```python
from build123d import *
from build123d.topology import SkipClean

# Parameters (mm, degrees)
SKETCH1_R                    = 4
COUPLER_SECTION_DEPTH        = 12.5
SKETCH3_R                    = 5
BEARING_SECTION_DEPTH        = 12
SKETCH4_R                    = 7
BEARING_STOP_DEPTH           = 3
SKETCH5_R                    = 4
SMALL_SEAL_SECTION_DEPTH     = 12.3
SET_SCREW_FLAT_SECTION_DEPTH = 10.5
SKETCH7_R                    = 4
IMPELLER_SECTION_DEPTH       = 15.35455
SKETCH8_R                    = 1.5
IMPELLER_BOLT_BORE_DEPTH     = 8
DOWEL_PIN_HOLE_DEPTH         = 23
DOWEL_PIN_HOLE_DEPTH_BACK    = 23
SKETCH9_R                    = 1


with BuildPart() as part:
    # Sketch1 → coupler section (new body)
    with BuildSketch(Plane(origin=(0, 0, 0), x_dir=(1, 0, 0), z_dir=(0, 1, 0))):
        with Locations(Location((0, 0, 0), (0, 0, 270))):
            Circle(SKETCH1_R)
    extrude(amount=COUPLER_SECTION_DEPTH)

    # Sketch3 → bearing section (add)
    with BuildSketch(Plane(origin=(0, 12.5, 0), x_dir=(1, 0, 0), z_dir=(0, 1, 0))):
        with Locations(Location((0, 0, 0), (0, 0, 270))):
            Circle(SKETCH3_R)
    extrude(amount=BEARING_SECTION_DEPTH)

    # Sketch4 → bearing stop (add)
    with BuildSketch(Plane(origin=(0, 24.5, 0), x_dir=(1, 0, 0), z_dir=(0, 1, 0))):
        with Locations(Location((0, 0, 0), (0, 0, 270))):
            Circle(SKETCH4_R)
    extrude(amount=BEARING_STOP_DEPTH)

    # Sketch5 → small seal section (add)
    with BuildSketch(Plane(origin=(0, 27.5, 0), x_dir=(1, 0, 0), z_dir=(0, 1, 0))):
        with Locations(Location((0, 0, 0), (0, 0, 270))):
            Circle(SKETCH5_R)
    extrude(amount=SMALL_SEAL_SECTION_DEPTH)

    # Sketch6 → set screw flat section (cut)
    with BuildSketch(Plane.XZ):
        with BuildLine():
            Line((-2.645751311, 3), (2.645751311, 3))
            ThreePointArc((2.645751311, 3), (0, 4), (-2.645751311, 3))
        make_face()
    extrude(amount=-SET_SCREW_FLAT_SECTION_DEPTH, mode=Mode.SUBTRACT)

    # Sketch7 → impeller section (add)
    with BuildSketch(Plane(origin=(0, 39.8, 0), x_dir=(1, 0, 0), z_dir=(0, 1, 0))):
        with Locations(Location((0, 0, 0), (0, 0, 311.409622109))):
            Circle(SKETCH7_R)
    extrude(amount=IMPELLER_SECTION_DEPTH)

    # Sketch8 → impeller bolt bore (cut)
    with BuildSketch(Plane(origin=(0, 55.15455, 0), x_dir=(1, 0, 0), z_dir=(0, 1, 0))):
        with Locations(Location((0, 0, 0), (0, 0, 270))):
            Circle(SKETCH8_R)
    extrude(amount=-IMPELLER_BOLT_BORE_DEPTH, mode=Mode.SUBTRACT)

    # Sketch9 → dowel pin hole (cut, two sides: drawn at the far end of the back side and taken through both)
    with SkipClean():  # the faces are left unmerged after this step: merging them gives an invalid solid
        with BuildSketch(Plane.XY.offset(-DOWEL_PIN_HOLE_DEPTH_BACK)):
            with Locations(Location((0, 44.15455, 0), (0, 0, 89.999999996))):
                Circle(SKETCH9_R)
        extrude(amount=DOWEL_PIN_HOLE_DEPTH + DOWEL_PIN_HOLE_DEPTH_BACK, mode=Mode.SUBTRACT)


solid = part.part
```
Geometry check sheet. Reference: the model listing, model coordinates, mm. A direction names the side the tool comes from. Round coordinates to 2 decimals unless told otherwise and drop trailing zeros. Order: outer loops, then holes, each group sorted by start corner. A loop starts at its lowest first (then second) coordinate and runs counter-clockwise, first axis right, second up. Notation, with made-up numbers: (-19.75, -18.75) - (29.25, -18.75) arc R21 cw to (29.25, -6.75) - close; hole circle Ø11 at (-19.75, 42.5). An arc over 180 degrees is marked (long way). Use a Markdown table: item, result. Add a question column.
(1) Sectioned sample at D-D, the plane z = -6. Enter the section's corners in (x, y).
(2) Depth check by flat-ended pin: pin 1 (2.5 mm diameter, centred on x = 0, y = 44.15, fed in from -Z); pin 2 (2.5 mm diameter, centred on x = 0, z = 0, fed in from +Y); pin 3 (6 mm diameter, centred on x = -0.5, y = 5.5, fed in from +Z). Enter the tip coordinate at first touch or a pass-through.
(3) Material ranges on line 1 along X through (y, z) = (50.5, 0); line 2 along Y through (x, z) = (6.25, 0); line 3 along Y through (x, z) = (-0.25, 3.5), recorded low to high. Write a range as [from, to].
(4) Tool access check on faces 1 (the cylindrical face through (-1.9, 41.13, 3.52)), 2 (the flat face through (0, 5, 3)), 3 (the cylindrical face through (-6.834, 25.979, -1.517)), 4 (the cylindrical face through (-4.88, 18.42, -1.08)). Record the directions out of +Z, -Z, +X, -X, +Y, -Y that give a thin tool (end or side, any length) a straight path to the whole face; none if there is none.
(5) Release check for a two-part mould opening along Y. For faces 5 (the cylindrical face through (0.38, 45.08, -0.06)), 6 (the flat face through (0, 0, -1)), 7 (the flat face through (0, 47.155, 0)) record: pulls with the +Y half, pulls with the -Y half, needs draft (parallel to the pull), parting line crosses it, or undercut.
(6) Sectioned sample at C-C, the plane y = 5. Enter the section's corners in (x, z), and give its area (3 significant figures).
(7) Sectioned sample at A-A, the plane z = 0. Enter the section's corners in (x, y).
(8) Sectioned sample at B-B, the plane x = -0.5. Enter the section's corners in (y, z).
Answers below:
| question | item | result |
|---|---|---|
| 1 | outline | (-3.61, 24.5) - (3.61, 24.5) - (3.61, 27.5) - (-3.61, 27.5) - close |
| 2 | pin 1 | z = -4 |
| 2 | pin 2 | y = 47.15 |
| 2 | pin 3 | z = 3 |
| 3 | line 1 | [-4, -1.5], [1.5, 4] |
| 3 | line 2 | [24.5, 27.5] |
| 3 | line 3 | [10.5, 43.19], [45.12, 55.15] |
| 4 | face 1 | +Y |
| 4 | face 2 | +Z, +X, -X, -Y |
| 4 | face 3 | +Y, -Y |
| 4 | face 4 | -Y |
| 5 | face 5 | undercut |
| 5 | face 6 | pulls with the -Y half |
| 5 | face 7 | pulls with the +Y half |
| 6 | outline | (-2.65, 3) arc R4 ccw (long way) to (2.65, 3) - close |
| 6 | area | 46.6 mm² |
| 7 | outline | (-7, 24.5) - (-5, 24.5) - (-5, 12.5) - (-4, 12.5) - (-4, 0) - (4, 0) - (4, 12.5) - (5, 12.5) - (5, 24.5) - (7, 24.5) - (7, 27.5) - (4, 27.5) - (4, 55.15) - (1.5, 55.15) - (1.5, 47.15) - (-1.5, 47.15) - (-1.5, 55.15) - (-4, 55.15) - (-4, 27.5) - (-7, 27.5) - close; hole circle Ø2 at (0, 44.15) |
| 8 | outline | (0, -3.97) - (12.5, -3.97) - (12.5, -4.97) - (24.5, -4.97) - (24.5, -6.98) - (27.5, -6.98) - (27.5, -3.97) - (43.29, -3.97) - (43.29, 3.97) - (27.5, 3.97) - (27.5, 6.98) - (24.5, 6.98) - (24.5, 4.97) - (12.5, 4.97) - (12.5, 3.97) - (10.5, 3.97) - (10.5, 3) - (0, 3) - close; (45.02, -3.97) - (55.15, -3.97) - (55.15, -1.41) - (47.15, -1.41) - (47.15, 1.41) - (55.15, 1.41) - (55.15, 3.97) - (45.02, 3.97) - close |
